The model under review builds one solid part; all positions refer to its coordinate system, in mm. Face numbers are marked on the shaded views. A direction names the side the tool comes from. Round coordinates to 2 decimals unless told otherwise and drop trailing zeros. Loops run counter-clockwise (first coordinate to the right, second up) from the corner with the lowest first, then second, coordinate; pieces in that order, holes last. Notation, with made-up numbers: M 68,12 L 97,12 A14 cw 97,20 Z; hole C -27.5,82 d1. An arc over 180 degrees is marked long. Use a Markdown table: item, result. Add a question column.
```python
from build123d import *

# Parameters (mm, degrees)
BOSS_EXTRUDE1_DEPTH = 29
SKETCH14_R          = 6
BOSS_EXTRUDE3_DEPTH = 28.45
SKETCH15_W          = 16
SKETCH15_H          = 12
BOSS_EXTRUDE4_DEPTH = 20.45
BOSS_EXTRUDE5_START = -12
BOSS_EXTRUDE5_DEPTH = 12
SKETCH17_R          = 6
CUT_EXTRUDE1_DEPTH  = 98.063123791


with BuildPart() as part:
    # Sketch1 → Boss-Extrude1 (new body)
    with BuildSketch(Plane.XY):
        with BuildLine():
            Line((-51, -30), (-19, -30))
            ThreePointArc((-19, -30), (-13.45, -35.55), (-19, -41.1))
            Line((-19, -41.1), (-51, -41.1))
            Line((-51, -41.1), (-51, -53.1))
            Line((-51, -53.1), (0, -53.1))
            Line((0, -53.1), (0, 0))
            Line((0, 0), (-32, 0))
            ThreePointArc((-32, 0), (-37.55, 5.55), (-32, 11.1))
            Line((-32, 11.1), (0, 11.1))
            Line((0, 11.1), (0, 23.1))
            Line((0, 23.1), (-51, 23.1))
            Line((-51, 23.1), (-51, -30))
        make_face()
    extrude(amount=BOSS_EXTRUDE1_DEPTH)

    # Sketch14 → Boss-Extrude3 (add)
    with BuildSketch(Plane(origin=(0, 23.1, 0), x_dir=(1, 0, 0), z_dir=(0, 1, 0))):
        with Locations(Location((-25.5, -14.5, 0), (0, 0, 180))):
            Circle(SKETCH14_R)
    boss_extrude3 = extrude(amount=BOSS_EXTRUDE3_DEPTH)

    # Sketch15 → Boss-Extrude4 (add)
    with BuildSketch(Plane(origin=(0, 51.55, 0), x_dir=(1, 0, 0), z_dir=(0, 1, 0))):
        with Locations((-25.5, -14.5)):
            Rectangle(SKETCH15_W, SKETCH15_H)
    boss_extrude4 = extrude(amount=BOSS_EXTRUDE4_DEPTH)

    # Sketch16 → Boss-Extrude5 (add)
    with BuildSketch(Plane.XY.offset(20.5).offset(BOSS_EXTRUDE5_START)):
        with BuildLine():
            Line((-17.5, 72), (-33.5, 72))
            ThreePointArc((-33.5, 72), (-25.5, 80), (-17.5, 72))
        make_face()
    boss_extrude5 = extrude(amount=BOSS_EXTRUDE5_DEPTH)

    # Sketch17 → Cut-Extrude1 (cut, through all)
    with BuildSketch(Plane.XY.offset(20.5)):
        with Locations((-25.5, 64)):
            Circle(SKETCH17_R)
    cut_extrude1 = extrude(amount=-CUT_EXTRUDE1_DEPTH, mode=Mode.SUBTRACT)

    # Mirror7: Boss-Extrude3, Boss-Extrude4, Boss-Extrude5, Cut-Extrude1 across plane
    add(boss_extrude3.mirror(Plane.ZX.offset(-15)))
    add(boss_extrude4.mirror(Plane.ZX.offset(-15)))
    add(boss_extrude5.mirror(Plane.ZX.offset(-15)))
    add(cut_extrude1.mirror(Plane.ZX.offset(-15)), mode=Mode.SUBTRACT)


solid = part.part
```
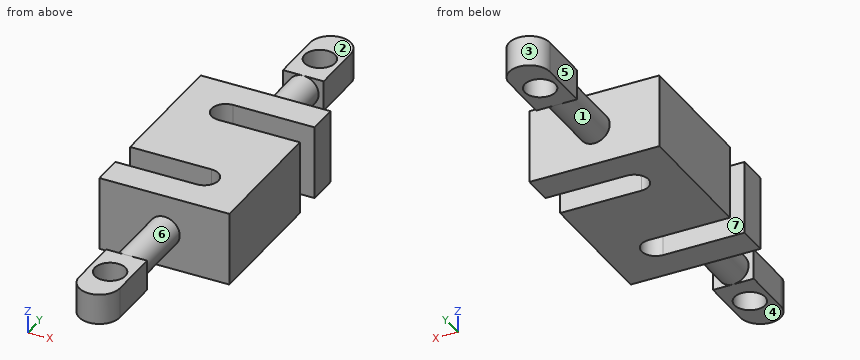
(1) Consider section B-B, the plane x = -47.5. Give the boundary of the cut face in (y, z).
(2) Draft analysis for pull direction Y (two halves, no side actions). For the marked faces 1, 2 and 3, state which applies: released by +Y, released by -Y, zero draft, split by the parting line, or undercut.
(3) Insertion check: pin 1 Ø10 at (x, z) = (-19, 22) entering from -Y; pin 2 Ø5 at (x, z) = (-8, 22) entering from +Y; pin 3 Ø4 at (y, z) = (-91, 17) entering from +X; pin 4 Ø9.5 at (x, y) = (-25.5, -94) entering from +Z. Each pin has a flat end and moves straight along its axis. Give the tip position at first contact, or say it passes through.
(4) To check wall thickness, follow probe 1 along Y at (x, z) = (-25.5, 12); probe 2 along X at (y, z) = (-94, 13); probe 3 along Y at (x, z) = (-6.5, 19.5). State the ranges of each line that lie inside material, in increasing order.
(5) For the marked faces 4, 5, 6 and 7, list the 3-axis set-ups (+Z, -Z, +X, -X, +Y, -Y) from which the entire face can be reached by the end or side of a thin tool; tool diameter is ignored.
(6) Consider section C-C, the plane z = 26.5. Give the boundary of the cut face in (x, y).
(7) Consider section D-D, the plane z = 14.5. Give the number of separate pieces and of enclosed holes in the cut face, then the cut area to 3 significant figures.
(8) Consider section A-A, the plane y = 64. Give the boundary of the cut face in (x, z), then the cut area to 3 significant figures.
Found:
| question | item | result |
|---|---|---|
| 1 | outline | M -53.1,0 L -41.1,0 L -41.1,29 L -53.1,29 Z; M -30,0 L 23.1,0 L 23.1,29 L -30,29 Z |
| 2 | face 1 | undercut |
| 2 | face 2 | zero draft |
| 2 | face 3 | released by +Y |
| 3 | pin 1 | stops at y = -109.81 |
| 3 | pin 2 | stops at y = 23.1 |
| 3 | pin 3 | stops at x = -17.5 |
| 3 | pin 4 | passes through |
| 4 | probe 1 | y = -110 to -100, -88 to -41.1, -30 to 0, 11.1 to 58, 70 to 80 |
| 4 | probe 2 | x = -33.5 to -31.5, -19.5 to -17.5 |
| 4 | probe 3 | y = -53.1 to 0, 11.1 to 23.1 |
| 5 | face 4 | -Z, +X, -X, -Y |
| 5 | face 5 | +Z, -Z, -X, +Y |
| 5 | face 6 | none |
| 5 | face 7 | +Z, -Z, -X |
| 6 | outline | M -51,-53.1 L 0,-53.1 L 0,0 L -32,0 A5.55 cw -32,11.1 L 0,11.1 L 0,23.1 L -51,23.1 L -51,-30 L -19,-30 A5.55 cw -19,-41.1 L -51,-41.1 Z |
| 7 | separate pieces | 1 |
| 7 | enclosed holes | 2 |
| 7 | area | 4,390 mm^2 |
| 8 | outline | M -33.5,8.5 L -31.5,8.5 L -31.5,20.5 L -33.5,20.5 Z; M -19.5,8.5 L -17.5,8.5 L -17.5,20.5 L -19.5,20.5 Z |
| 8 | area | 48.0 mm^2 |
